from build123d import *

# Parameters (mm, degrees)
SKETCH_1_W               = 36
SKETCH_1_H               = 8
EXTRUDE_1_DEPTH          = 11
SKETCH_2_W               = 8
SKETCH_2_H               = 8
SKETCH_2_W_2             = 12
CUT_EXTRUDE_1_DEPTH      = 9
FILLET_1_R               = 4
CUT_EXTRUDE_2_DEPTH      = 28.586228448
CUT_EXTRUDE_2_DEPTH_BACK = 28.586228448
SKETCH_3_R               = 1.5
FILLET_2_R               = 2
CUT_EXTRUDE_3_DEPTH      = 9


with BuildPart() as part:
    # 草图1 → 凸台-拉伸1 (new body)
    with BuildSketch(Plane.XY):
        with Locations((18, -4)):
            Rectangle(SKETCH_1_W, SKETCH_1_H)
    extrude(amount=EXTRUDE_1_DEPTH)

    # 草图2 → 切除-拉伸1 (cut)
    with BuildSketch(Plane.XY.offset(11)):
        with Locations((18, -4)):
            Rectangle(SKETCH_2_W, SKETCH_2_H)
        with Locations((6, -4)):
            Rectangle(SKETCH_2_W_2, SKETCH_2_H)
        with Locations((30, -4)):
            Rectangle(SKETCH_2_W_2, SKETCH_2_H)
    extrude(amount=-CUT_EXTRUDE_1_DEPTH, mode=Mode.SUBTRACT)

    # 圆角1
    fillet_1_edges = [part.edges().sort_by_distance(p)[0] for p in [
        (23, -8, 11),
        (23, 0, 11),
        (13, 0, 11),
        (13, -8, 11),
    ]]
    fillet(fillet_1_edges, radius=FILLET_1_R - 0.0001)  # a hair under: the kernel refuses the full size

    # 草图3 → 切除-拉伸2 (cut, two sides: drawn at the far end of the back side and taken through both)
    with BuildSketch(Plane.ZY.offset(-12).offset(-CUT_EXTRUDE_2_DEPTH_BACK)):
        with Locations((7.5, -4)):
            Circle(SKETCH_3_R)
    extrude(amount=CUT_EXTRUDE_2_DEPTH + CUT_EXTRUDE_2_DEPTH_BACK, mode=Mode.SUBTRACT)

    # 圆角2
    fillet_2_edges = [part.edges().sort_by_distance(p)[0] for p in [
        (0, -8, 1),
        (0, 0, 1),
        (36, 0, 1),
        (36, -8, 1),
    ]]
    fillet(fillet_2_edges, radius=FILLET_2_R)

    # 草图4 → 切除-拉伸3 (cut)
    with BuildSketch(Plane.XY.offset(2)):
        with BuildLine():
            Line((32, -2.5), (26.5, -2.5))
            ThreePointArc((26.5, -2.5), (25, -4), (26.5, -5.5))
            Line((26.5, -5.5), (32, -5.5))
            ThreePointArc((32, -5.5), (33.5, -4), (32, -2.5))
        make_face()
        with BuildLine():
            Line((4, -2.5), (9.5, -2.5))
            ThreePointArc((9.5, -2.5), (11, -4), (9.5, -5.5))
            Line((9.5, -5.5), (4, -5.5))
            ThreePointArc((4, -5.5), (2.5, -4), (4, -2.5))
        make_face()
    extrude(amount=-CUT_EXTRUDE_3_DEPTH, mode=Mode.SUBTRACT)


solid = part.part
Geometry: final body of the model. Coordinates: model frame, mm. A direction names the side the tool comes from. Round coordinates to 2 decimals unless told otherwise and drop trailing zeros. Write each loop counter-clockwise with the first axis right and the second up, starting at its lowest first coordinate (ties: lowest second). Pieces come first, ordered by that corner, then holes. Notation, with made-up numbers: M -29,-1 L 7,-1 A28 cw 7,22 Z; hole C 4,-13 d3. An arc over 180 degrees is marked long. Write item = value, one per line.
Item 1: Section query A-A on x = 29. Return loops of the section in (y, z), then the cut area to 3 significant figures.
Findings:
outline = M -8,0 L -5.5,0 L -5.5,2 L -8,2 Z; M -2.5,0 L 0,0 L 0,2 L -2.5,2 Z
area = 10.0 mm^2
Item 2: Access query for faces 1 (the face through (14, -4.1, 5.6)), 2 (the face through (29, -2.5, 1)), 3 (the face through (36, -4, 1)). Directions: +Z, -Z, +X, -X, +Y, -Y. A direction counts if a zero-diameter tool reaches every point of the face in a straight line with its end or side. Return the directions, or none.
Findings:
face_1 = +Z, +Y, -Y
face_2 = +Z, -Z
face_3 = +Z, -Z, +X, +Y, -Y
Item 3: Pull-direction query (X, two-part tool) for faces 4 (the face through (13.014, -1.141, 9.797)), 5 (the face through (25, -4, 1)), 6 (the face through (12, -4.1, 5.6)); classes: pulls with the +X half, pulls with the -X half, needs draft (parallel to the pull), parting line crosses it, or undercut.
Findings:
face_4 = needs draft
face_5 = undercut
face_6 = pulls with the -X half
Item 4: Pin query (flat end, axial travel): P1, Ø3, axis at y = -4.5, z = 6, coming from the -X side; P2, Ø1.5, axis at x = 28.5, y = -7, coming from the +Z side; P3, Ø4, axis at x = 11.5, y = -6.5, coming from the +Z side; P4, Ø2.5, axis at y = -4, z = 7.5, coming from the +X side. Return the tip coordinate at first contact, or that it passes through.
Findings:
P1 = 12
P2 = 2
P3 = 10.96
P4 = through
Item 5: Section query B-B on z = 4. Return loops of the section in (x, y), then the cut area to 3 significant figures.
Findings:
outline = M 12,-8 L 14,-8 L 14,0 L 12,0 Z; M 22,-8 L 24,-8 L 24,0 L 22,0 Z
area = 32.0 mm^2
Item 6: Section query D-D on z = 7.75. Return loops of the section in (x, y).
Findings:
outline = M 12,-7.93 L 14,-7.93 L 14,-5.48 L 12,-5.48 Z; M 12,-2.52 L 14,-2.52 L 14,-0.07 L 12,-0.07 Z; M 22,-7.93 L 24,-7.93 L 24,-5.48 L 22,-5.48 Z; M 22,-2.52 L 24,-2.52 L 24,-0.07 L 22,-0.07 Z
Item 7: Section query C-C on y = -3.5. Return loops of the section in (x, z), then the cut area to 3 significant figures.
Findings:
outline = M 0,0 L 2.59,0 L 2.59,2 L 0,2 Z; M 10.91,0 L 25.09,0 L 25.09,2 L 24,2 L 24,6.09 L 22,6.09 L 22,2 L 14,2 L 14,6.09 L 12,6.09 L 12,2 L 10.91,2 Z; M 12,8.91 L 14,8.91 L 14,10.97 L 12,10.97 Z; M 22,8.91 L 24,8.91 L 24,10.97 L 22,10.97 Z; M 33.41,0 L 36,0 L 36,2 L 33.41,2 Z
area = 63.2 mm^2
Item 8: Material intervals for line 1 along Y through (x, z) = (31, 1.5); line 2 along Z through (x, y) = (22.7, -4); line 3 along X through (y, z) = (-2.75, 8.75), sorted ascending. Write a range as [from, to].
Findings:
line_1 = [-8, -5.5], [-2.5, 0]
line_2 = [0, 6], [9, 11]
line_3 = [12, 14], [22, 24]
